Could you check a few things on this model? Use its own coordinates, in mm. Face numbers are marked on the shaded views. A direction names the side the tool comes from. Give positions to 0.01 mm unless a question says otherwise; leave off trailing zeros. Order: outer loops, then holes, each group sorted by start corner. A loop starts at its lowest first (then second) coordinate and runs counter-clockwise, first axis right, second up. Notation, with made-up numbers: M 10.25,-21 L 49.25,-21 A30 cw 49.25,17 Z; hole C 57.5,83.5 d8. An arc over 180 degrees is marked long. Use a Markdown table: item, result. Add a question column.
```python
from build123d import *

# Parameters (mm, degrees)
SKETCH_1_W           = 48.51
SKETCH_1_H           = 34
SKETCH_1_W_2         = 28.51
SKETCH_1_H_2         = 14
EXTRUDE_1_DEPTH      = 12.25
SKETCH_2_R           = 1.91
CUT_EXTRUDE_1_DEPTH  = 33.05257439
SKETCH_4_W           = 13
SKETCH_4_H           = 13.91
EXTRUDE_1_2_DEPTH    = 74.82
SKETCH_5_W           = 13.91
SKETCH_5_H           = 16.23
EXTRUDE_2_DEPTH      = 15
SKETCH_7_R           = 24.5
SKETCH_7_R_2         = 14.5
EXTRUDE_2_2_DEPTH    = 16.23
SKETCH_12_R          = 1.9
CUT_EXTRUDE_4_DEPTH  = 97.312124675
EXTRUDE_3_DEPTH      = 10
EXTRUDE_3_DEPTH_BACK = 8
SKETCH_13_W          = 13.91
SKETCH_13_H          = 16.23
SKETCH_14_R          = 1.9
CUT_EXTRUDE_5_DEPTH  = 103.744583434


with BuildPart() as part:
    # 草圖1 → Extrude 1 (new body)
    with BuildSketch(Plane(origin=(0, 0, 0), x_dir=(1, 0, 0), z_dir=(0, 1, 0))):
        Rectangle(SKETCH_1_W, SKETCH_1_H)
        Rectangle(SKETCH_1_W_2, SKETCH_1_H_2, mode=Mode.SUBTRACT)
    extrude(amount=EXTRUDE_1_DEPTH)

    # 草圖2 → 除料-伸長1 (cut, through all)
    with BuildSketch(Plane(origin=(0, 12.25, 0), x_dir=(1, 0, 0), z_dir=(0, 1, 0))):
        with Locations(Location((-19.255, 0, 0), (0, 0, 270))):
            Circle(SKETCH_2_R)
        with Locations(Location((19.255, 0, 0), (0, 0, 270))):
            Circle(SKETCH_2_R)
    extrude(amount=-CUT_EXTRUDE_1_DEPTH, mode=Mode.SUBTRACT)

    # 草圖4 → Extrude 1 2 (add)
    with BuildSketch(Plane.XZ):
        with Locations((17.755, 0)):
            Rectangle(SKETCH_4_W, SKETCH_4_H)
    extrude(amount=EXTRUDE_1_2_DEPTH)

    # 草圖5 → Extrude 2 (add)
    with BuildSketch(Plane.ZY.offset(-11.255)):
        with Locations((0, -66.705)):
            Rectangle(SKETCH_5_W, SKETCH_5_H)
    extrude(amount=EXTRUDE_2_DEPTH)

    # 草圖7 → Extrude 2 2 (add)
    with BuildSketch(Plane(origin=(3.626674765, -74.82, 0), x_dir=(1, 0, 0), z_dir=(0, -1, 0))):
        with Locations((-30.978154344, 0)):
            Circle(SKETCH_7_R)
        with Locations((-30.978154344, 0)):
            Circle(SKETCH_7_R_2, mode=Mode.SUBTRACT)
    extrude(amount=-EXTRUDE_2_2_DEPTH)

    # 草圖12 → 除料-伸長4 (cut, through all)
    with BuildSketch(Plane(origin=(0, 0, -6.955), x_dir=(-1, 0, 0), z_dir=(0, 0, -1))):
        with Locations((-3.856713649, -66.705)):
            Circle(SKETCH_12_R)
    extrude(amount=-CUT_EXTRUDE_4_DEPTH, mode=Mode.SUBTRACT)

    # 草圖13 → 填料-伸長3 (add, two sides: drawn at the far end of the back side and taken through both)
    with BuildSketch(Plane(origin=(-55, 0, 0), x_dir=(0, 0, -1), z_dir=(1, 0, 0)).offset(-EXTRUDE_3_DEPTH_BACK)):
        with Locations((0, -66.705)):
            Rectangle(SKETCH_13_W, SKETCH_13_H)
    extrude(amount=EXTRUDE_3_DEPTH + EXTRUDE_3_DEPTH_BACK)

    # 草圖14 → 除料-伸長5 (cut, through all)
    with BuildSketch(Plane(origin=(0, 0, -6.955), x_dir=(-1, 0, 0), z_dir=(0, 0, -1))):
        with Locations((56.908040017, -66.705)):
            Circle(SKETCH_14_R)
    extrude(amount=-CUT_EXTRUDE_5_DEPTH, mode=Mode.SUBTRACT)


solid = part.part
```
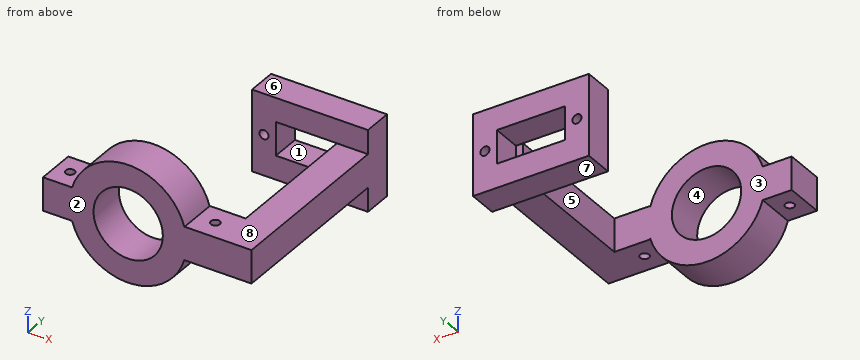
1) Please list where these lines run through material, in increasing order: line 1 (X direction, y = 2.75, z = 0) (3 decimals); line 2 (Y direction, x = -9, z = 1); line 3 (Y direction, x = 3, z = 5.5). Write a range as from..to.
2) Suppose I cut it at C-C on y = 6. Please give me the cut outline in (x, z) (3 decimals).
3) Suppose I cut it at D-D on y = -38. Please give me the cut outline in (x, z) (3 decimals), and give its area (3 significant figures).
4) Suppose I cut it at A-A on z = 0. Please give me the cut outline in (x, y) (3 decimals).
5) Suppose I cut it at B-B on x = -29.5. Please give me the cut outline in (y, z).
6) We'd pull the mould along Y, two halves only. Please class the marked faces 1, 2 and 3: pulls with the +Y half, pulls with the -Y half, needs draft (parallel to the pull), parting line crosses it, or undercut.
7) For the marked faces 4, 5, 6, 7 and 8, which set-ups out of +Z, -Z, +X, -X, +Y, -Y let a thin tool reach every point of the face, with its end or its side?
8) For pin 1 (10 mm diameter, centred on x = -13, y = -4, fed in from +Z); pin 2 (13.5 mm diameter, centred on x = 6, y = 3.5, fed in from -Z); pin 3 (3.5 mm diameter, centred on x = -57, y = -69, fed in from -Z) (3 decimals), each with a flat end and sliding along its axis, tell me the tip position at first contact or that it passes through.
Values found:
| question | item | result |
|---|---|---|
| 1 | line 1 | x = -24.255..-21.165, -17.345..-14.255, 14.255..17.345, 21.165..24.255 |
| 1 | line 2 | y = -74.82..-58.59 |
| 1 | line 3 | y = -74.82..-68.4, -65.01..-58.59 |
| 2 | outline | M -24.255,-17 L 24.255,-17 L 24.255,17 L -24.255,17 Z; hole C -19.255,0 d3.82; hole M -14.255,-7 L 14.255,-7 L 14.255,7 L -14.255,7 Z; hole C 19.255,0 d3.82 |
| 3 | outline | M 11.255,-6.955 L 24.255,-6.955 L 24.255,6.955 L 11.255,6.955 Z |
| 3 | area | 181 mm^2 |
| 4 | outline | M -63,-74.82 L -41.851,-74.82 L -41.851,-58.59 L -63,-58.59 Z; M -24.255,0 L -21.165,0 L -21.165,12.25 L -24.255,12.25 Z; M -17.345,0 L -14.255,0 L -14.255,12.25 L -17.345,12.25 Z; M -12.851,-74.82 L 24.255,-74.82 L 24.255,12.25 L 21.165,12.25 L 21.165,0 L 17.345,0 L 17.345,12.25 L 14.255,12.25 L 14.255,0 L 11.255,0 L 11.255,-58.59 L -12.851,-58.59 Z; hole C -56.908,-66.705 d3.8; hole C 3.857,-66.705 d3.8 |
| 5 | outline | M -74.82,-24.41 L -58.59,-24.41 L -58.59,-14.34 L -74.82,-14.34 Z; M -74.82,14.34 L -58.59,14.34 L -58.59,24.41 L -74.82,24.41 Z |
| 6 | face 1 | needs draft |
| 6 | face 2 | pulls with the -Y half |
| 6 | face 3 | undercut |
| 7 | face 4 | -Y |
| 7 | face 5 | +Z, -Z, -X, +Y |
| 7 | face 6 | +Z, +X, -X, +Y |
| 7 | face 7 | -Z, +X, -X, +Y |
| 7 | face 8 | +Z, +X, -Y |
| 8 | pin 1 | stops at z = 17 |
| 8 | pin 2 | stops at z = -17 |
| 8 | pin 3 | stops at z = -6.955 |
